For this review, take the finished solid that the model builds, in its own axes (mm). A direction names the side the tool comes from. Give positions to 0.01 mm unless a question says otherwise; leave off trailing zeros. Write each loop counter-clockwise with the first axis right and the second up, starting at its lowest first coordinate (ties: lowest second). Pieces come first, ordered by that corner, then holes.
Q1. We need section B-B (z = 0). Write out the cut boundary in (x, y).
Q2. Machinability: for faces 4 (the cylindrical face through (-3.955, 0.493, -5.158)), 5 (the cylindrical face through (-3.955, 5.507, -5.158)), 6 (the flat face through (-6, 6, 4)), which of the approach directions +Z, -Z, +X, -X, +Y, -Y give a long, thin tool a straight path to every point of the face, cutting with its end or side? Answer none if there is none.
Q3. We need section C-C (y = 5.4). Write out the cut boundary in (x, z), then the cut area to 3 significant figures.
Q4. Mouldability with a two-part tool opening along Z and no side actions: class faces 1 (the flat face through (-6, 0, 4)), 2 (the flat face through (-1, 5, 3)), 3 (the cylindrical face through (-5.78, 2.96, -7.54)) as released by +Z, released by -Z, zero draft, split by the parting line, or undercut.
Q5. We need section D-D (x = -4). Write out the cut boundary in (y, z), then the cut area to 3 significant figures.
Q6. Insertion check: P1, Ø10, axis at x = 2.5, z = -5.5, coming from the +Y side; P2, Ø9.5, axis at x = 0, z = 0, coming from the +Y side; P3, Ø1, axis at y = 3.5, z = 4, coming from the +X side; P4, Ø1, axis at y = 0.5, z = 6, coming from the -X side. Each pin has a flat end and moves straight along its axis. Give the tip position at first contact, or say it passes through.
Q7. We need section A-A (x = 0). Write out the cut boundary in (y, z), then the cut area to 3 significant figures.
Q8. For line 1 (X direction, y = 0.6, z = 0); line 2 (X direction, y = 2.4, z = 0); line 3 (Z direction, x = -3.5, y = 5.3), list the stretches that pass through material, from the lowest coordinate up.
```python
from build123d import *

# Parameters (mm, degrees)
SKETCH1_R           = 9.5
BOSS_EXTRUDE1_DEPTH = 6
SKETCH2_R           = 6.5
CUT_EXTRUDE1_DEPTH  = 1
SKETCH3_R           = 3
CUT_EXTRUDE2_DEPTH  = 15.335271187


with BuildPart() as part:
    # Sketch1 → Boss-Extrude1 (new body)
    with BuildSketch(Plane(origin=(0, 0, 0), x_dir=(1, 0, 0), z_dir=(0, 1, 0))):
        with Locations(Location((0, 0, 0), (0, 0, 270))):
            Circle(SKETCH1_R)
    extrude(amount=BOSS_EXTRUDE1_DEPTH)

    # Sketch2 → Cut-Extrude1 (cut)
    with BuildSketch(Plane(origin=(0, 6, 0), x_dir=(1, 0, 0), z_dir=(0, 1, 0))):
        with Locations(Location((0, 0, 0), (0, 0, 270))):
            Circle(SKETCH2_R)
    cut_extrude1 = extrude(amount=-CUT_EXTRUDE1_DEPTH, mode=Mode.SUBTRACT)

    # Sketch3 → Cut-Extrude2 (cut, through all)
    with BuildSketch(Plane(origin=(0, 5, 0), x_dir=(1, 0, 0), z_dir=(0, 1, 0))):
        with Locations(Location((0, 0, 0), (0, 0, 270))):
            Circle(SKETCH3_R)
    extrude(amount=-CUT_EXTRUDE2_DEPTH, mode=Mode.SUBTRACT)

    # Mirror1: Cut-Extrude1 across plane
    add(cut_extrude1.mirror(Plane.ZX.offset(3)), mode=Mode.SUBTRACT)


solid = part.part
```
Computed:
1. outline: (-9.5, 0) - (-6.5, 0) - (-6.5, 1) - (-3, 1) - (-3, 5) - (-6.5, 5) - (-6.5, 6) - (-9.5, 6) - close; (3, 1) - (6.5, 1) - (6.5, 0) - (9.5, 0) - (9.5, 6) - (6.5, 6) - (6.5, 5) - (3, 5) - close
2. face 4: -Y
2. face 5: +Y
2. face 6: +Z, -Z, +X, -X, +Y
3. outline: circle Ø19 at (0, 0); hole circle Ø13 at (0, 0)
3. area: 151 mm2
4. face 1: zero draft
4. face 2: undercut
4. face 3: split by the parting line
5. outline: (0, -8.62) - (6, -8.62) - (6, -5.12) - (5, -5.12) - (5, 5.12) - (6, 5.12) - (6, 8.62) - (0, 8.62) - (0, 5.12) - (1, 5.12) - (1, -5.12) - (0, -5.12) - close
5. area: 82.9 mm2
6. P1: stops at y = 6
6. P2: stops at y = 5
6. P3: stops at x = 8.83
6. P4: stops at x = -7.75
7. outline: (0, -9.5) - (6, -9.5) - (6, -6.5) - (5, -6.5) - (5, -3) - (1, -3) - (1, -6.5) - (0, -6.5) - close; (0, 6.5) - (1, 6.5) - (1, 3) - (5, 3) - (5, 6.5) - (6, 6.5) - (6, 9.5) - (0, 9.5) - close
7. area: 64.0 mm2
8. line 1: x = -9.5 to -6.5, 6.5 to 9.5
8. line 2: x = -9.5 to -3, 3 to 9.5
8. line 3: z = -8.83 to -5.48, 5.48 to 8.83
